CAD build for the part. Positions are in the model's coordinates, mm. A direction names the side the tool comes from. Give positions to 0.01 mm unless a question says otherwise; leave off trailing zeros. Order: outer loops, then holes, each group sorted by start corner. A loop starts at its lowest first (then second) coordinate and runs counter-clockwise, first axis right, second up. Notation, with made-up numbers: (9.25, 68) -> (40.25, 68) arc R26 cw to (40.25, 96) -> close; hole circle Ø10 at (42, 52). An arc over 180 degrees is marked (long way). Use one line per item in the form item = value. Start each with the question number.
1) Tool access for faces 1 (the face through (-20, 17, -2)), 2 (the face through (-32, 15, 0)), 3 (the face through (20.35, 34, -2)), 4 (the face through (-14.327, 15.226, 7.957)): list every direction of +Z, -Z, +X, -X, +Y, -Y with a clear straight run to the whole face (end or side of a thin tool).
2) Probe line 1 (X direction, y = 27, z = 3); line 2 (X direction, y = 15, z = 2); line 3 (Z direction, x = -11.5, y = 34). List the from-to ranges inside material, lowest first.
3) Drop flat-ended pins along their axis: P1, Ø3.5, axis at x = 15.5, y = 32.5, coming from the +Z side; P2, Ø3.5, axis at x = 24, z = 2.5, coming from the +Y side; P3, Ø1.5, axis at x = -1, y = 33.5, coming from the +Z side. Give the stop position or say it passes through.
4) Cut at A-A, the plane y = 22. Give the cut face in (x, z), and give its area (3 significant figures).
5) Cut at C-C, the plane z = 17.5. Give the cut face in (x, y).
6) Cut at D-D, the plane z = -8. Give the cut face in (x, y).
7) Mould opens along Z. For faces 5 (the face through (-10.65, 15.23, 9.68)), 6 (the face through (-3.906, 31, 0)), 7 (the face through (25.586, 15.274, 2.292)) say: pulls with the +Z half, pulls with the -Z half, needs draft (parallel to the pull), parting line crosses it, or undercut.
8) Cut at B-B, the plane x = -7. Give the cut face in (y, z), and give its area (3 significant figures).
from build123d import *
from build123d.topology import SkipClean

# Parameters (mm, degrees)
CROQUIS1_W              = 70
CROQUIS1_H              = 65
EXTRUIR1_DEPTH          = 3.5
CROQUIS2_R              = 3.1
EXTRUIR2_DEPTH          = 5
EXTRUIR3_DEPTH          = 10
CROQUIS4_OUTSIDE_W      = 91.294
CROQUIS4_OUTSIDE_H      = 86.294
EXTRUIR4_DEPTH          = 10
REDONDEO1_R             = 3
EXTRUIR5_DEPTH          = 13.5
EXTRUIR6_DEPTH          = 3.5
CROQUIS7_R              = 1.6
EXTRUIR7_DEPTH          = 47.982330447
CROQUIS8_R              = 3.1
EXTRUIR8_DEPTH          = 5
CROQUIS9_W              = 0.7
CROQUIS9_H              = 10.5
EXTRUIR9_DEPTH          = 10
EXTRUIR10_DEPTH         = 63.752948337
EXTRUIR10_DEPTH_BACK    = 10
CROQUIS10_W             = 3.0625
CROQUIS10_H             = 5
SALIENTE_EXTRUIR1_DEPTH = 4
SALIENTE_EXTRUIR2_DEPTH = 20
CROQUIS14_R             = 1.5
CORTAR_EXTRUIR2_DEPTH   = 65


with BuildPart() as part:
    # Croquis1 → Extruir1 (new body)
    with BuildSketch(Plane(origin=(0, 0, 0), x_dir=(1, 0, 0), z_dir=(0, 1, 0))):
        Rectangle(CROQUIS1_W, CROQUIS1_H)
    extrude(amount=EXTRUIR1_DEPTH)

    # Croquis2 → Extruir2 (cut)
    with BuildSketch(Plane(origin=(0, 3.5, 0), x_dir=(1, 0, 0), z_dir=(0, 1, 0))):
        with Locations(Location((0, -17.5, 0), (0, 0, 270))):
            Circle(CROQUIS2_R)
    extrude(amount=-EXTRUIR2_DEPTH, mode=Mode.SUBTRACT)

    # Croquis3 → Extruir3 (add)
    with BuildSketch(Plane(origin=(0, 3.5, 0), x_dir=(1, 0, 0), z_dir=(0, 1, 0))):
        with BuildLine():
            Line((-34.4868, 13.5), (20.3496, 13.5))
            Line((20.3496, 13.5), (20.3496, 0))
            Line((20.3496, 0), (17.146428199, 0))
            ThreePointArc((17.146428199, 0), (22.955777517, -8.939493087), (24.418230894, -19.5))
            Line((24.418230894, -19.5), (9.287087811, -19.5))
            ThreePointArc((9.287087811, -19.5), (-3.635492607, -26.276855559), (-7.981176331, -12.347250794))
            Line((-7.981176331, -12.347250794), (-18.680510212, -1.647916913))
            ThreePointArc((-18.680510212, -1.647916913), (-17.932408832, -0.806327142), (-17.146428199, 0))
            Line((-17.146428199, 0), (-34.4868, 0))
            Line((-34.4868, 0), (-34.4868, 13.5))
        make_face()
        with BuildLine():
            Line((-32.9868, 1.5), (-12.961481397, 1.5))
            ThreePointArc((-12.961481397, 1.5), (-14.868021343, 0.048274597), (-16.613165932, -1.593940849))
            Line((-16.613165932, -1.593940849), (-5.999348286, -12.207758495))
            ThreePointArc((-5.999348286, -12.207758495), (-3.061467459, -24.89103626), (7.984359711, -18))
            Line((7.984359711, -18), (22.994564575, -18))
            ThreePointArc((22.994564575, -18), (20.451694563, -6.977253708), (12.961481397, 1.5))
            Line((12.961481397, 1.5), (18.8496, 1.5))
            Line((18.8496, 1.5), (18.8496, 12))
            Line((18.8496, 12), (-32.9868, 12))
            Line((-32.9868, 12), (-32.9868, 1.5))
        make_face(mode=Mode.SUBTRACT)
    extrude(amount=EXTRUIR3_DEPTH)

    # Croquis4 outside → Extruir4 (cut)
    with SkipClean():  # the faces are left unmerged after this step: merging them gives an invalid solid
        with BuildSketch(Plane(origin=(0, 3.5, 0), x_dir=(1, 0, 0), z_dir=(0, 1, 0))):
            Rectangle(CROQUIS4_OUTSIDE_W, CROQUIS4_OUTSIDE_H)
            with BuildLine():
                Line((-34.4868, 0), (-17.146428199, 0))
                ThreePointArc((-17.146428199, 0), (-17.932408832, -0.806327142), (-18.680510212, -1.647916913))
                Line((-18.680510212, -1.647916913), (-7.981176331, -12.347250794))
                ThreePointArc((-7.981176331, -12.347250794), (-3.635492607, -26.276855559), (9.287087811, -19.5))
                Line((9.287087811, -19.5), (24.418230894, -19.5))
                ThreePointArc((24.418230894, -19.5), (22.955777517, -8.939493087), (17.146428199, 0))
                Line((17.146428199, 0), (20.3496, 0))
                Line((20.3496, 0), (20.3496, 13.5))
                Line((20.3496, 13.5), (-34.4868, 13.5))
                Line((-34.4868, 13.5), (-34.4868, 0))
            make_face(mode=Mode.SUBTRACT)
        extrude(amount=-EXTRUIR4_DEPTH, mode=Mode.SUBTRACT)

    # Redondeo1
    redondeo1_edges = [part.edges().sort_by_distance(p)[0] for p in [
        (-7.981176331, 8.5, 12.347250794),
        (9.287087811, 8.5, 19.5),
        (-5.999348286, 8.5, 12.207758495),
        (7.984359711, 8.5, 18),
    ]]
    fillet(redondeo1_edges, radius=REDONDEO1_R)

    # Croquis5 → Extruir5 (add)
    with SkipClean():  # the faces are left unmerged after this step: merging them gives an invalid solid
        with BuildSketch(Plane.XZ):
            with BuildLine():
                Line((-18.680510212, 1.647916913), (-14.437869525, 5.8905576))
                ThreePointArc((-14.437869525, 5.8905576), (-21.723092903, 6.819250451), (-24.449770984, 0))
                Line((-24.449770984, 0), (-17.146428199, 0))
                ThreePointArc((-17.146428199, 0), (-17.932408832, 0.806327142), (-18.680510212, 1.647916913))
            make_face()
            with BuildLine():
                Line((20.3496, 0), (20.3496, -13.5))
                ThreePointArc((20.3496, -13.5), (28.665212431, 2.225567304), (24.418230894, 19.5))
                ThreePointArc((24.418230894, 19.5), (22.955777517, 8.939493087), (17.146428199, 0))
                Line((17.146428199, 0), (20.3496, 0))
            make_face()
        extrude(amount=-EXTRUIR5_DEPTH)

    # Chaflán1
    # the kernel refuses this chamfer: 5, 4.044665138 mm, written as the material it adds along each edge
    with BuildSketch(Plane(origin=(-14.437869525, 3.5, 5.8905576), x_dir=(-0.8768595348589333, 0, 0.4807466652270976), z_dir=(0, 1, 0))) as chafl_n1_piece_1:
        with BuildLine():
            Line((2.949791971, 0), (-1.211824758, 3.780414953))
            Line((-1.211824758, 3.780414953), (-1.307822013, 3.752405544))
            ThreePointArc((-1.307822013, 3.752405544), (-0.651776703, 1.876825504), (-0.095997255, -0.02800941))
            Line((-0.095997255, -0.02800941), (0.02800941, -0.095997255))
            ThreePointArc((0.02800941, -0.095997255), (1.47002525, 0.136406993), (2.931105495, -0.098238565))
            Line((2.931105495, -0.098238565), (2.949791971, 0))
        make_face()
    extrude(amount=10)
    with BuildSketch(Plane(origin=(-24.449770984, 3.5, 0), x_dir=(-0.008036803743584595, 0, 0.9999677043712897), z_dir=(0, 1, 0))) as chafl_n1_piece_2:
        with BuildLine():
            Line((2.423263449, 0), (-0.064845869, -4.38542071))
            Line((-0.064845869, -4.38542071), (-0.164842639, -4.386224391))
            ThreePointArc((-0.164842639, -4.386224391), (-0.082377051, -2.193111839), (-0.09999677, -0.00080368))
            Line((-0.09999677, -0.00080368), (0.026691621, 0.096371974))
            ThreePointArc((0.026691621, 0.096371974), (1.204598314, -0.104316531), (2.411212242, 0.099271186))
            Line((2.411212242, 0.099271186), (2.423263449, 0))
        make_face()
    extrude(amount=10)
    with BuildSketch(Plane(origin=(-24.449770984, 0, 0), x_dir=(-0.9997395779240649, 0, -0.022820524363231526), z_dir=(0, 1, 0))) as chafl_n1_piece_3:
        with BuildLine():
            Line((4.385900112, 0), (-0.035828136, 2.422998574))
            Line((-0.035828136, 2.422998574), (-0.134910293, 2.409480951))
            ThreePointArc((-0.134910293, 2.409480951), (0.08649505, 1.206008973), (-0.096756078, 0.025263837))
            Line((-0.096756078, 0.025263837), (0.002282052, -0.099973958))
            ThreePointArc((0.002282052, -0.099973958), (2.194090072, -0.04994272), (4.388182164, -0.099973958))
            Line((4.388182164, -0.099973958), (4.385900112, 0))
        make_face()
    extrude(amount=3.5)
    with BuildSketch(Plane(origin=(-14.437869525, 0, 5.8905576), x_dir=(0.7254657554746632, 0, 0.6882582637597433), z_dir=(0, 1, 0))) as chafl_n1_piece_4:
        with BuildLine():
            Line((3.96989376, 0), (-0.900434913, -2.809001538))
            Line((-0.900434913, -2.809001538), (-0.98828054, -2.761219262))
            ThreePointArc((-0.98828054, -2.761219262), (-0.318834214, -1.441501248), (-0.099965384, 0.002630967))
            Line((-0.099965384, 0.002630967), (0.002630967, 0.099965384))
            ThreePointArc((0.002630967, 0.099965384), (1.986203869, 0.047760165), (3.972524727, 0.099965384))
            Line((3.972524727, 0.099965384), (3.96989376, 0))
        make_face()
    extrude(amount=3.5)


with BuildPart() as body_2:
    # Croquis6 → Extruir6 (new body)
    with BuildSketch(Plane(origin=(0, 13.5, 0), x_dir=(1, 0, 0), z_dir=(0, 1, 0))):
        with BuildLine():
            Line((-34.4868, 13.5), (-34.4868, 0))
            Line((-34.4868, 0), (-28.661374979, 0))
            Line((-28.661374979, 0), (-24.642400208, -2.323096648))
            ThreePointArc((-24.642400208, -2.323096648), (-21.929637735, -6.692039268), (-16.829963308, -7.355409896))
            Line((-16.829963308, -7.355409896), (-11.752306982, -8.576120143))
            Line((-11.752306982, -8.576120143), (-9.515139435, -10.813287689))
            ThreePointArc((-9.515139435, -10.813287689), (-8.69974084, -12.321679102), (-8.843709432, -14.030302105))
            ThreePointArc((-8.843709432, -14.030302105), (-3.635492607, -26.276855559), (8.70689382, -21.3))
            ThreePointArc((8.70689382, -21.3), (9.813271565, -19.99001992), (11.456439237, -19.5))
            Line((11.456439237, -19.5), (24.418230894, -19.5))
            ThreePointArc((24.418230894, -19.5), (28.665212431, -2.225567304), (20.3496, 13.5))
            Line((20.3496, 13.5), (-34.4868, 13.5))
        make_face()
    extrude(amount=EXTRUIR6_DEPTH)


with BuildPart() as extruir7_tool:
    # Croquis7 → Extruir7 (new, through all)
    with BuildSketch(Plane(origin=(0, 17, 0), x_dir=(1, 0, 0), z_dir=(0, 1, 0))):
        with Locations(Location((-20, -2.5, 0), (0, 0, 270))):
            Circle(CROQUIS7_R)
        with Locations(Location((24, -2.5, 0), (0, 0, 270))):
            Circle(CROQUIS7_R)
    extrude(amount=-EXTRUIR7_DEPTH)


with BuildPart() as part_1:
    add(part.part)

    # Extruir7: cut by extruir7_tool
    add(extruir7_tool.part, mode=Mode.SUBTRACT)

    # Croquis9 → Extruir9 (cut)
    with BuildSketch(Plane(origin=(0, 13.5, 0), x_dir=(1, 0, 0), z_dir=(0, 1, 0))):
        with Locations((19.1996, 6.75)):
            Rectangle(CROQUIS9_W, CROQUIS9_H)
    extrude(amount=-EXTRUIR9_DEPTH, mode=Mode.SUBTRACT)

    # Croquis10 → Extruir10 (cut, two sides: drawn at the far end of the back side and taken through both)
    with BuildSketch(Plane.ZY.offset(-19.5496).offset(-EXTRUIR10_DEPTH_BACK)):
        with Locations((-8.9375, 8.5)):
            Rectangle(CROQUIS10_W, CROQUIS10_H)
    extrude(amount=EXTRUIR10_DEPTH + EXTRUIR10_DEPTH_BACK, mode=Mode.SUBTRACT)


with BuildPart() as body_2_1:
    add(body_2.part)

    # Extruir7: cut by extruir7_tool
    add(extruir7_tool.part, mode=Mode.SUBTRACT)

    # Croquis8 → Extruir8 (cut)
    with BuildSketch(Plane(origin=(0, 17, 0), x_dir=(1, 0, 0), z_dir=(0, 1, 0))):
        with Locations(Location((0, -17.5, 0), (0, 0, 270))):
            Circle(CROQUIS8_R)
    extrude(amount=-EXTRUIR8_DEPTH, mode=Mode.SUBTRACT)

    # Croquis11 → Saliente-Extruir1 (add)
    with BuildSketch(Plane(origin=(0, 0, -13.5), x_dir=(-1, 0, 0), z_dir=(0, 0, -1))):
        Polygon((34.4868, 17), (34.4868, 38.05596306), (-20.3496, 50.212900258), (-20.3496, 17), align=None)
    extrude(amount=-SALIENTE_EXTRUIR1_DEPTH)

    # Croquis13 → Saliente-Extruir2 (add)
    with BuildSketch(Plane.XY.offset(-9.5)):
        Polygon((-10.905631326, 43.283782293), (-3.905631326, 44.835644932), (-3.905631326, 17), (-10.905631326, 17), align=None)
        Polygon((20.3496, 50.212900258), (13.3496, 48.66103762), (13.3496, 17), (20.3496, 17), align=None)
    extrude(amount=SALIENTE_EXTRUIR2_DEPTH)

    # Croquis14 → Cortar-Extruir2 (cut)
    with BuildSketch(Plane.XY.offset(10.5)):
        with Locations((-7.405631326, 30.64159382)):
            Circle(CROQUIS14_R)
        with Locations((16.8496, 33.23257477)):
            Circle(CROQUIS14_R)
    extrude(amount=-CORTAR_EXTRUIR2_DEPTH, mode=Mode.SUBTRACT)


solid = body_2_1.part
Result:
q1.face_1 = +Z, -X, +Y
q1.face_2 = +Z, -X, +Y, -Y
q1.face_3 = +Z, -Z, +X, +Y
q1.face_4 = +Z, +Y, -Y
q2.line_1 = -10.91 to -3.91, 13.35 to 20.35
q2.line_2 = -25.2 to -21.52, -18.48 to 22.48, 25.52 to 28.64
q2.line_3 = -13.5 to -9.5
q3.P1 = 10.5
q3.P2 = 17
q3.P3 = -9.5
q4.outline = (-34.49, -13.5) -> (20.35, -13.5) -> (20.35, 10.5) -> (13.35, 10.5) -> (13.35, -9.5) -> (-3.91, -9.5) -> (-3.91, 10.5) -> (-10.91, 10.5) -> (-10.91, -9.5) -> (-34.49, -9.5) -> close
q4.area = 499 mm²
q5.outline = (-9.5, 13.5) -> (-3.1, 13.5) -> (-3.1, 17) -> (-9.5, 17) -> close; (3.1, 13.5) -> (25.67, 13.5) -> (25.67, 17) -> (3.1, 17) -> close
q6.outline = (-34.49, 13.5) -> (25.03, 13.5) -> (25.03, 17) -> (20.35, 17) -> (20.35, 50.21) -> (13.35, 48.66) -> (13.35, 17) -> (-3.91, 17) -> (-3.91, 44.84) -> (-10.91, 43.28) -> (-10.91, 17) -> (-34.49, 17) -> close; hole circle Ø3 at (-7.41, 30.64); hole circle Ø3 at (16.85, 33.23)
q7.face_5 = pulls with the +Z half
q7.face_6 = needs draft
q7.face_7 = undercut
q8.outline = (13.5, -13.5) -> (29.2, -13.5) -> (29.2, 10.5) -> (17, 10.5) -> (17, 23.92) -> (13.5, 23.92) -> close; (32.09, -13.5) -> (44.15, -13.5) -> (44.15, 10.5) -> (32.09, 10.5) -> close
q8.area = 713 mm²
